Autodesk Inventor part; units mm, degrees
ref_plane "YZ Plane" through (0, 0, 0) normal (1, 0, 0) x (0, 1, 0)
ref_plane "XZ Plane" through (0, 0, 0) normal (0, 1, 0) x (-1, 0, 0)
ref_plane "XY Plane" through (0, 0, 0) normal (0, 0, 1) x (1, 0, 0)
sketch "Sketch1" plane through (0, 0, 0) normal (0, 0, 1) x (1, 0, 0)
  line L0 (32.1184, 271.7487) -> (82.1184, 271.7487)
  line L1 (82.1184, 271.7487) -> (82.1184, 21.7487)
  line L2 (82.1184, 21.7487) -> (32.1184, 21.7487)
  line L3 (32.1184, 21.7487) -> (32.1184, 271.7487)
  point P0 (0, 0)
  dimension "d0" = 50
  dimension "d1" = 250
extrude "Extrusion1" add sketch "Sketch1" along normal blind 5
sketch "Sketch2" plane through (0, 0, 5) normal (0, 0, 1) x (1, 0, 0)
  line L0 (82.1184, 271.7487) -> (32.1184, 271.7487)
  line L1 (57.1184, 271.7487) -> (47.1184, 271.7487)
  line L2 (47.1184, 271.7487) -> (47.1184, 276.7487)
  line L3 (47.1184, 276.7487) -> (67.1184, 276.7487)
  line L4 (67.1184, 276.7487) -> (67.1184, 271.7487)
  line L5 (32.1184, 21.7487) -> (82.1184, 21.7487)
  line L6 (32.1184, 21.7487) -> (32.1184, 16.7487)
  line L7 (32.1184, 16.7487) -> (47.1184, 16.7487)
  line L8 (47.1184, 16.7487) -> (47.1184, 21.7487)
  line L9 (82.1184, 21.7487) -> (82.1184, 16.7487)
  line L10 (82.1184, 16.7487) -> (67.1184, 16.7487)
  line L11 (67.1184, 16.7487) -> (67.1184, 21.7487)
  point P0 (0, 0)
  dimension "d4" = 10
  dimension "d5" = 5
  dimension "d6" = 20
  dimension "d7" = 5
  dimension "d8" = 15
  dimension "d9" = 5
  dimension "d10" = 15
extrude "Extrusion2" add sketch "Sketch2" against normal blind 5 contours L0 L2 L3 L4
sketch "Sketch3" plane through (0, 0, 5) normal (0, 0, 1) x (1, 0, 0)
  line L0 (32.1184, 21.7487) -> (82.1184, 21.7487)
  line L1 (32.1184, 21.7487) -> (32.1184, 16.7487)
  line L2 (32.1184, 16.7487) -> (47.1184, 16.7487)
  line L3 (47.1184, 16.7487) -> (47.1184, 21.7487)
  line L4 (82.1184, 21.7487) -> (82.1184, 16.7487)
  line L5 (82.1184, 16.7487) -> (67.1184, 16.7487)
  line L6 (67.1184, 16.7487) -> (67.1184, 21.7487)
  point P0 (0, 0)
  dimension "d13" = 5
  dimension "d14" = 15
  dimension "d15" = 5
  dimension "d16" = 15
extrude "Extrusion3" add sketch "Sketch3" against normal blind 5
sketch "Sketch4" plane through (0, 0, 5) normal (0, 0, 1) x (1, 0, 0)
  line L0 (47.1184, 21.7487) -> (67.1184, 21.7487)
  line L1 (57.1184, 21.7487) -> (57.1184, 26.7487)
  line L2 (57.1184, 26.7487) -> (47.1184, 26.7487)
  line L3 (47.1184, 26.7487) -> (47.1184, 21.7487)
  line L4 (47.1184, 21.7487) -> (67.1184, 21.7487)
  line L5 (67.1184, 21.7487) -> (67.1184, 26.7487)
  line L6 (67.1184, 26.7487) -> (57.1184, 26.7487)
  line L7 (47.1184, 21.7487) -> (32.1184, 21.7487)
  line L8 (32.1184, 21.7487) -> (82.1184, 21.7487)
  line L9 (82.1184, 16.7487) -> (82.1184, 271.7487)
  point P0 (0, 0)
  dimension "d19" = 5
  dimension "d20" = 10
  dimension "d21" = 15
sketch "Sketch5" plane through (0, 0, 5) normal (0, 0, 1) x (1, 0, 0)
  point P0 (0, 0)
sketch "Sketch6" plane through (0, 0, 5) normal (0, 0, 1) x (1, 0, 0)
  line L0 (47.1184, 21.7487) -> (67.1184, 21.7487)
  line L1 (47.1184, 21.7487) -> (47.1184, 16.7487)
  line L2 (47.1184, 21.7487) -> (47.1184, 16.7487)
  line L3 (32.1184, 271.7487) -> (32.1184, 16.7487)
  line L4 (47.1184, 16.7487) -> (32.1184, 16.7487)
  line L5 (32.1184, 16.7487) -> (32.1184, 21.7487)
  line L6 (47.1184, 21.7487) -> (32.1184, 21.7487)
  line L7 (32.1184, 21.7487) -> (32.1184, 16.7487)
  line L8 (32.1184, 16.7487) -> (47.1184, 16.7487)
  point P0 (0, 0)
extrude "Extrusion4" cut sketch "Sketch6" against normal blind 15
extrude "Extrusion5" cut sketch "Sketch4" against normal blind 15
sketch "Sketch7" plane through (0, 0, 5) normal (0, 0, 1) x (1, 0, 0)
  line L0 (67.1184, 26.7487) -> (67.1184, 16.7487)
  line L1 (67.1184, 21.7487) -> (67.1184, 16.7487)
  line L2 (82.1184, 16.7487) -> (82.1184, 271.7487)
  line L3 (67.1184, 16.7487) -> (82.1184, 16.7487)
  line L4 (82.1184, 16.7487) -> (82.1184, 21.7487)
  line L5 (67.1184, 21.7487) -> (82.1184, 21.7487)
  point P0 (0, 0)
extrude "Extrusion6" cut sketch "Sketch7" against normal blind 15
sketch "Sketch8" plane through (0, 0, 5) normal (0, 0, 1) x (1, 0, 0)
  line L0 (47.1184, 276.7487) -> (67.1184, 276.7487)
  line L1 (57.1184, 276.7487) -> (57.1184, 26.7487)
  line L2 (67.1184, 26.7487) -> (47.1184, 26.7487)
  point P0 (0, 0)
sketch "Sketch9" plane through (0, 0, 5) normal (0, 0, 1) x (1, 0, 0)
  line L0 (47.1184, 276.7487) -> (67.1184, 276.7487)
  line L1 (57.1184, 276.7487) -> (57.1184, 26.7487)
  line L2 (67.1184, 26.7487) -> (47.1184, 26.7487)
  line L3 (67.1184, 21.7487) -> (67.1184, 26.7487)
  line L4 (67.1184, 26.7487) -> (67.1184, 21.7487)
  line L5 (82.1184, 271.7487) -> (82.1184, 21.7487)
  line L6 (67.1184, 21.7487) -> (82.1184, 21.7487)
  line L7 (82.1184, 21.7487) -> (82.1184, 271.7487)
  line L8 (82.1184, 271.7487) -> (67.1184, 271.7487)
  line L9 (67.1184, 271.7487) -> (67.1184, 276.7487)
  line L10 (67.1184, 276.7487) -> (57.1184, 276.7487)
  line L11 (67.1184, 276.7487) -> (67.1184, 271.7487)
  point P0 (0, 0)
extrude "Extrusion7" cut sketch "Sketch9" against normal blind 15
equation "\"d22\" = d21"
equation "\"d24\" = d21"
equation "\"d26\" = d21"
equation "\"d28\" = d21"
properties material "Steel, Carbon"
For this review, take the finished solid that the model builds, in its own axes (mm). A direction names the side the tool comes from. Round coordinates to 2 decimals unless told otherwise and drop trailing zeros. Write each loop counter-clockwise with the first axis right and the second up, starting at its lowest first coordinate (ties: lowest second). Pieces come first, ordered by that corner, then holes. Notation, with made-up numbers: (48, 0.25) -> (95, 0.25) arc R38 ccw to (95, 38.25) -> close; hole circle Ø9 at (2.25, 4.5). An arc over 180 degrees is marked (long way). Put each result on its own line as item: value.
Q1. Consider section A-A on z = 1.6. State the section outline as (x, y) points.
Determined:
outline: (32.12, 21.75) -> (47.12, 21.75) -> (47.12, 26.75) -> (57.12, 26.75) -> (57.12, 276.75) -> (47.12, 276.75) -> (47.12, 271.75) -> (32.12, 271.75) -> close
Q2. Consider section B-B on x = 52. State the section outline as (y, z) points, and give its area (3 significant figures).
Determined:
outline: (26.75, 0) -> (276.75, 0) -> (276.75, 5) -> (26.75, 5) -> close
area: 1,250 mm^2
Q3. To check wall thickness, follow L1, parallel to Y at x = 36.5, z = 4.4; L2, parallel to Y at x = 52.25, z = 2.05. State the ranges of each line that lie inside material, in increasing order. Write a range as [from, to].
Determined:
L1: y = [21.75, 271.75]
L2: y = [26.75, 276.75]
Q4. Machinability: for faces 1 (the flat face through (47.118, 274, 3)), 2 (the flat face through (47.118, 24, 3)), 3 (the flat face through (57.118, 153, 3)), which of the approach directions +Z, -Z, +X, -X, +Y, -Y give a long, thin tool a straight path to every point of the face, cutting with its end or side? Answer none if there is none.
Determined:
face 1: +Z, -Z, -X, +Y
face 2: +Z, -Z, +X, -Y
face 3: +Z, -Z, +X, +Y, -Y
Q5. Clearance check with flat-ended pins moving along their axes: pin 1 Ø1.5 at (x, z) = (54, 3) entering from -Y; pin 2 Ø1.5 at (x, z) = (45.5, 0.5) entering from +Y; pin 3 Ø2.5 at (y, z) = (275, 2.5) entering from -X. State where each tip first meets the part, or that it passes through.
Determined:
pin 1: stops at y = 26.75
pin 2: stops at y = 271.75
pin 3: stops at x = 47.12
